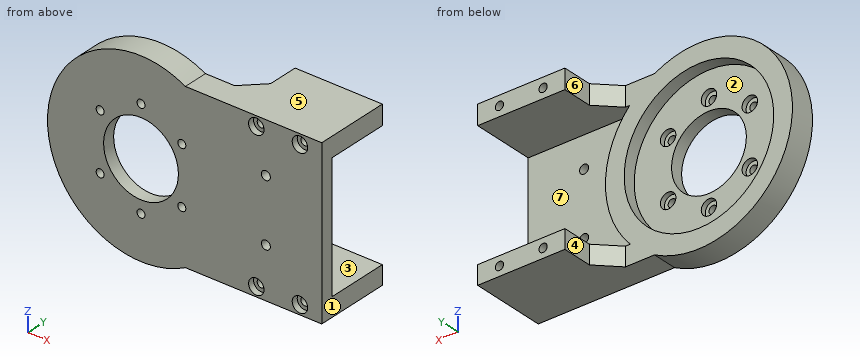
from build123d import *

# Parameters (mm, degrees)
SKETCH1_R                            = 37.5
SKETCH1_R_2                          = 15
BOSS_EXTRUDE2_DEPTH                  = 5
SKETCH3_R                            = 37.5
SKETCH3_R_2                          = 30
BOSS_EXTRUDE3_DEPTH                  = 5
SKETCH4_R                            = 1.6
CUT_EXTRUDE1_DEPTH                   = 5
SKETCH5_R                            = 3.1
CUT_EXTRUDE2_DEPTH                   = 2
BOSS_EXTRUDE4_DEPTH                  = 35
BOSS_EXTRUDE4_DIRECTION_2_REACH      = 86.447
BOSS_EXTRUDE4_DIRECTION_2_END_RADIUS = 37.5
SKETCH9_W                            = 35
SKETCH9_H                            = 7.85
SKETCH9_H_2                          = 7.55
BOSS_EXTRUDE5_DEPTH                  = 20.2
CHAMFER1_SIZE                        = 8
SKETCH11_R                           = 1.65
CUT_EXTRUDE3_DEPTH                   = 88.031833257
SKETCH12_R                           = 3.1
CUT_EXTRUDE4_DEPTH                   = 2.5
SKETCH15_R                           = 1.8
CUT_EXTRUDE5_DEPTH                   = 10


with BuildPart() as part:
    # Sketch1 → Boss-Extrude2 (new body)
    with BuildSketch(Plane(origin=(0, 0, 0), x_dir=(1, 0, 0), z_dir=(0, 1, 0))):
        with Locations(Location((0, 0, 0), (0, 0, 270))):
            Circle(SKETCH1_R)
        with Locations(Location((0, 0, 0), (0, 0, 270))):
            Circle(SKETCH1_R_2, mode=Mode.SUBTRACT)
    extrude(amount=BOSS_EXTRUDE2_DEPTH)

    # Sketch3 → Boss-Extrude3 (add)
    with BuildSketch(Plane(origin=(0, 5, 0), x_dir=(1, 0, 0), z_dir=(0, 1, 0))):
        with Locations(Location((0, 0, 0), (0, 0, 270))):
            Circle(SKETCH3_R)
        with Locations(Location((0, 0, 0), (0, 0, 270))):
            Circle(SKETCH3_R_2, mode=Mode.SUBTRACT)
    extrude(amount=BOSS_EXTRUDE3_DEPTH)

    # Sketch4 → Cut-Extrude1 (cut)
    with BuildSketch(Plane(origin=(0, 5, 0), x_dir=(1, 0, 0), z_dir=(0, 1, 0))):
        with Locations(Location((0, 20, 0), (0, 0, 270))):
            Circle(SKETCH4_R)
        with Locations(Location((-16.383040886, 11.471528727, 0), (0, 0, 270))):
            Circle(SKETCH4_R)
        with Locations(Location((16.383040886, 11.471528727, 0), (0, 0, 270))):
            Circle(SKETCH4_R)
        with Locations(Location((16.383040886, -11.471528727, 0), (0, 0, 90))):
            Circle(SKETCH4_R)
        with Locations(Location((0, -20, 0), (0, 0, 90))):
            Circle(SKETCH4_R)
        with Locations(Location((-16.383040886, -11.471528727, 0), (0, 0, 90))):
            Circle(SKETCH4_R)
    extrude(amount=-CUT_EXTRUDE1_DEPTH, mode=Mode.SUBTRACT)

    # Sketch5 → Cut-Extrude2 (cut)
    with BuildSketch(Plane(origin=(0, 5, 0), x_dir=(1, 0, 0), z_dir=(0, 1, 0))):
        with Locations(Location((0, 20, 0), (0, 0, 270))):
            Circle(SKETCH5_R)
        with Locations(Location((-16.383040886, 11.471528727, 0), (0, 0, 270))):
            Circle(SKETCH5_R)
        with Locations(Location((16.383040886, 11.471528727, 0), (0, 0, 270))):
            Circle(SKETCH5_R)
        with Locations(Location((16.383040886, -11.471528727, 0), (0, 0, 90))):
            Circle(SKETCH5_R)
        with Locations(Location((-16.383040886, -11.471528727, 0), (0, 0, 90))):
            Circle(SKETCH5_R)
        with Locations(Location((0, -20, 0), (0, 0, 90))):
            Circle(SKETCH5_R)
    extrude(amount=-CUT_EXTRUDE2_DEPTH, mode=Mode.SUBTRACT)

    # Sketch8 → Boss-Extrude4 (add)
    with BuildSketch(Plane(origin=(37.5, 0, 0), x_dir=(0, 0, -1), z_dir=(1, 0, 0))):
        Polygon((33, 0), (33, 10), (25.45, 10), (25.45, 5), (-25.15, 5), (-25.15, 10), (-33, 10), (-33, 0), align=None)
    extrude(amount=BOSS_EXTRUDE4_DEPTH)

    # Boss-Extrude4 direction 2: up to this cylinder (the profile starts outside it)
    boss_extrude4_direction_2_end = Plane(origin=(0, 3.445946, 0), z_dir=(0, -1, 0)) * Cylinder(BOSS_EXTRUDE4_DIRECTION_2_END_RADIUS, 248.894, mode=Mode.PRIVATE)
    # Sketch8 → Boss-Extrude4 direction 2 (add, up to the surface)
    with BuildSketch(Plane(origin=(37.5, 0, 0), x_dir=(0, 0, -1), z_dir=(1, 0, 0)), mode=Mode.PRIVATE) as boss_extrude4_direction_2_sk1:
        Polygon((33, 0), (33, 10), (25.45, 10), (25.45, 5), (-25.15, 5), (-25.15, 10), (-33, 10), (-33, 0), align=None)
    boss_extrude4_direction_2_tool1 = extrude(boss_extrude4_direction_2_sk1.sketch, amount=-BOSS_EXTRUDE4_DIRECTION_2_REACH, mode=Mode.PRIVATE) - boss_extrude4_direction_2_end
    add(boss_extrude4_direction_2_tool1.solids().sort_by_distance((37.5, 3.445946, 0.093243))[0])
    add(boss_extrude4_direction_2_tool1.solids().sort_by_distance((37.5, 3.445946, 0.093243))[1])

    # Sketch9 → Boss-Extrude5 (add)
    with BuildSketch(Plane(origin=(0, 10, 0), x_dir=(1, 0, 0), z_dir=(0, 1, 0))):
        with Locations((55, -29.075)):
            Rectangle(SKETCH9_W, SKETCH9_H)
        with Locations((55, 29.225)):
            Rectangle(SKETCH9_W, SKETCH9_H_2)
    extrude(amount=BOSS_EXTRUDE5_DEPTH)

    # Chamfer1
    chamfer1_edges = [part.edges().sort_by_distance(p)[0] for p in [
        (37.5, 10, 29.075),
        (37.5, 10, -29.225),
    ]]
    chamfer(chamfer1_edges, length=CHAMFER1_SIZE)

    # Sketch11 → Cut-Extrude3 (cut, through all)
    with BuildSketch(Plane(origin=(0, 30.2, 0), x_dir=(1, 0, 0), z_dir=(0, 1, 0))):
        with Locations(Location((46.25, 29.225, 0), (0, 0, 270))):
            Circle(SKETCH11_R)
        with Locations(Location((63.75, 29.225, 0), (0, 0, 270))):
            Circle(SKETCH11_R)
        with Locations(Location((63.75, -29.075, 0), (0, 0, 270))):
            Circle(SKETCH11_R)
        with Locations(Location((46.25, -29.075, 0), (0, 0, 270))):
            Circle(SKETCH11_R)
    extrude(amount=-CUT_EXTRUDE3_DEPTH, mode=Mode.SUBTRACT)

    # Sketch12 → Cut-Extrude4 (cut)
    with BuildSketch(Plane.XZ):
        with Locations(Location((46.25, 29.075, 0), (0, 0, 270))):
            Circle(SKETCH12_R)
        with Locations(Location((63.75, 29.075, 0), (0, 0, 270))):
            Circle(SKETCH12_R)
        with Locations(Location((63.75, -29.225, 0), (0, 0, 270))):
            Circle(SKETCH12_R)
        with Locations(Location((46.25, -29.225, 0), (0, 0, 270))):
            Circle(SKETCH12_R)
    extrude(amount=-CUT_EXTRUDE4_DEPTH, mode=Mode.SUBTRACT)

    # Sketch15 → Cut-Extrude5 (cut)
    with BuildSketch(Plane(origin=(0, 5, 0), x_dir=(1, 0, 0), z_dir=(0, 1, 0))):
        with Locations(Location((50.089797686, 12.65, 0), (0, 0, 270))):
            Circle(SKETCH15_R)
        with Locations(Location((50.089797686, -12.65, 0), (0, 0, 270))):
            Circle(SKETCH15_R)
    extrude(amount=-CUT_EXTRUDE5_DEPTH, mode=Mode.SUBTRACT)


solid = part.part
Verification items for the finished model (mm, model axes). Face numbers are marked on the shaded views. A direction names the side the tool comes from. Coordinates: 2 decimals unless noted, no trailing zeros. Order: outer loops, then holes, each group sorted by start corner. A loop starts at its lowest first (then second) coordinate and runs counter-clockwise, first axis right, second up. Notation, with made-up numbers: (71, 22) -> (114, 22) arc R19 cw to (114, 42) -> close; hole circle Ø2 at (17.25, 75.25). An arc over 180 degrees is marked (long way). Put each result on its own line as item: value. Start each with the question number.
1. Material ranges on L1, parallel to Z at x = 49, y = 15; L2, parallel to X at y = 3, z = 30; L3, parallel to Z at x = 59.5, y = 2.5, recorded low to high. Write a range as [from, to].
2. Access from +Z, -Z, +X, -X, +Y, -Y to the whole of each face (thin tool, end or side, straight path). Record for the marked faces 5, 6 and 7.
3. Cross-section at C-C, the plane x = 46.25. Record the boundary of the cut face in (y, z) (3 decimals).
4. Mould release check, pull along X, two halves, no side actions. Record for the marked faces 1, 2, 3 and 4: released by +X, released by -X, zero draft, split by the parting line, or undercut.
5. Cross-section at D-D, the plane y = 24.5. Record the boundary of the cut face in (x, z) (3 decimals), then the cut area to 3 significant figures.
6. Cross-section at A-A, the plane y = 13.5. Record the boundary of the cut face in (x, z) (3 decimals).
7. Cross-section at B-B, the plane z = 0. Record the boundary of the cut face in (x, y).
8. Go/stop test with flat-tipped pins: pin 1 Ø5 at (x, y) = (-2.5, 8) entering from +Z; pin 2 Ø6 at (x, y) = (13.5, 12.5) entering from +Z; pin 3 Ø8 at (y, z) = (19.5, -22) entering from -X; pin 4 Ø10 at (y, z) = (6.5, -2) entering from +X. Record where each tip stops, or that it passes through.
Computed:
1. L1: [-33, -25.45], [25.15, 33]
1. L2: [-22.5, 44.88], [47.62, 62.38], [65.12, 72.5]
1. L3: [-33, 33]
2. face 5: +Z, +X, +Y, -Y
2. face 6: +Z, -Z, -X, +Y
2. face 7: +X, +Y
3. outline: (0, -33) -> (30.2, -33) -> (30.2, -30.875) -> (2.5, -30.875) -> (2.5, -32.325) -> (0, -32.325) -> close; (0, -26.125) -> (2.5, -26.125) -> (2.5, -27.575) -> (30.2, -27.575) -> (30.2, -25.45) -> (5, -25.45) -> (5, 25.15) -> (30.2, 25.15) -> (30.2, 27.425) -> (2.5, 27.425) -> (2.5, 25.975) -> (0, 25.975) -> close; (0, 32.175) -> (2.5, 32.175) -> (2.5, 30.725) -> (30.2, 30.725) -> (30.2, 33) -> (0, 33) -> close
4. face 1: released by +X
4. face 2: undercut
4. face 3: zero draft
4. face 4: released by -X
5. outline: (37.5, -33) -> (72.5, -33) -> (72.5, -25.45) -> (37.5, -25.45) -> close; (37.5, 25.15) -> (72.5, 25.15) -> (72.5, 33) -> (37.5, 33) -> close; hole circle Ø3.3 at (46.25, -29.225); hole circle Ø3.3 at (46.25, 29.075); hole circle Ø3.3 at (63.75, -29.225); hole circle Ø3.3 at (63.75, 29.075)
5. area: 505 mm2
6. outline: (33, -33) -> (72.5, -33) -> (72.5, -25.45) -> (33, -25.45) -> close; (33, 25.15) -> (72.5, 25.15) -> (72.5, 33) -> (33, 33) -> close; hole circle Ø3.3 at (46.25, -29.225); hole circle Ø3.3 at (46.25, 29.075); hole circle Ø3.3 at (63.75, -29.225); hole circle Ø3.3 at (63.75, 29.075)
7. outline: (-37.5, 0) -> (-15, 0) -> (-15, 5) -> (-30, 5) -> (-30, 10) -> (-37.5, 10) -> close; (15, 0) -> (72.5, 0) -> (72.5, 5) -> (37.5, 5) -> (37.5, 10) -> (30, 10) -> (30, 5) -> (15, 5) -> close
8. pin 1: z = 37.5
8. pin 2: z = 35.58
8. pin 3: x = 36.98
8. pin 4: x = 72.5
